```python
from build123d import *
from build123d.topology import SkipClean

# Parameters (mm, degrees)
ESQUISSE1_R        = 8
BOSS_EXTRU_1_DEPTH = 4.9
BOSS_EXTRU_2_START = 1.5
BOSS_EXTRU_2_DEPTH = 1.5
BOSS_EXTRU_3_DEPTH = 5


with BuildPart() as part:
    # Esquisse1 → Boss.-Extru.1 (new body)
    with BuildSketch(Plane.XY):
        with Locations((-10.25, -10)):
            Circle(ESQUISSE1_R)
        with BuildLine():
            Line((-5.751675839, -9.877200395), (-6.833750507, -9.782531128))
            Line((-6.833750507, -9.782531128), (-6.949445107, -9.126394451))
            Line((-6.949445107, -9.126394451), (-5.953521963, -8.661987862))
            ThreePointArc((-5.953521963, -8.661987862), (-6.006634107, -8.502052772), (-6.065697468, -8.344218516))
            Line((-6.065697468, -8.344218516), (-7.138261768, -8.631611254))
            Line((-7.138261768, -8.631611254), (-7.47139109, -8.054614344))
            Line((-7.47139109, -8.054614344), (-6.678798898, -7.262022153))
            ThreePointArc((-6.678798898, -7.262022153), (-6.782621037, -7.131675902), (-6.891198054, -7.005263035))
            Line((-6.891198054, -7.005263035), (-7.818046533, -7.654249327))
            Line((-7.818046533, -7.654249327), (-8.328430264, -7.225986526))
            Line((-8.328430264, -7.225986526), (-7.847635402, -6.194918616))
            ThreePointArc((-7.847635402, -6.194918616), (-7.988951343, -6.109285545), (-8.133315872, -6.028898352))
            Line((-8.133315872, -6.028898352), (-8.791112727, -6.968329619))
            Line((-8.791112727, -6.968329619), (-9.417191057, -6.740455742))
            Line((-9.417191057, -6.740455742), (-9.317216173, -5.597737589))
            ThreePointArc((-9.317216173, -5.597737589), (-9.478728542, -5.566588183), (-9.641271425, -5.541362369))
            Line((-9.641271425, -5.541362369), (-9.940094206, -6.656584169))
            Line((-9.940094206, -6.656584169), (-10.606352849, -6.656584169))
            Line((-10.606352849, -6.656584169), (-10.903477232, -5.547700874))
            ThreePointArc((-10.903477232, -5.547700874), (-11.065761738, -5.574558464), (-11.226956242, -5.607329229))
            Line((-11.226956242, -5.607329229), (-11.126406846, -6.756614081))
            Line((-11.126406846, -6.756614081), (-11.752485176, -6.984487958))
            Line((-11.752485176, -6.984487958), (-12.406540122, -6.050400691))
            ThreePointArc((-12.406540122, -6.050400691), (-12.550096477, -6.132241451), (-12.690551241, -6.219297732))
            Line((-12.690551241, -6.219297732), (-12.206963835, -7.256354271))
            Line((-12.206963835, -7.256354271), (-12.717347566, -7.684617071))
            Line((-12.717347566, -7.684617071), (-13.638885709, -7.039349117))
            ThreePointArc((-13.638885709, -7.039349117), (-13.74618945, -7.166864047), (-13.848697947, -7.298264801))
            Line((-13.848697947, -7.298264801), (-13.051434053, -8.095528695))
            Line((-13.051434053, -8.095528695), (-13.384563375, -8.672525605))
            Line((-13.384563375, -8.672525605), (-14.450903238, -8.3868007))
            ThreePointArc((-14.450903238, -8.3868007), (-14.508366703, -8.545244687), (-14.559856563, -8.705729393))
            Line((-14.559856563, -8.705729393), (-13.557961929, -9.172920534))
            Line((-13.557961929, -9.172920534), (-13.673656528, -9.829057211))
            Line((-13.673656528, -9.829057211), (-14.74934404, -9.923167674))
            ThreePointArc((-14.74934404, -9.923167674), (-14.749021481, -10.093838761), (-14.74222728, -10.264374865))
            Line((-14.74222728, -10.264374865), (-13.665452724, -10.358580432))
            Line((-13.665452724, -10.358580432), (-13.549758125, -11.014717109))
            Line((-13.549758125, -11.014717109), (-14.506309194, -11.460764198))
            ThreePointArc((-14.506309194, -11.460764198), (-14.447094307, -11.623083293), (-14.381691786, -11.78300953))
            Line((-14.381691786, -11.78300953), (-13.360941463, -11.509500306))
            Line((-13.360941463, -11.509500306), (-13.027812142, -12.086497216))
            Line((-13.027812142, -12.086497216), (-13.758807936, -12.817493011))
            ThreePointArc((-13.758807936, -12.817493011), (-13.646852578, -12.951506829), (-13.529782028, -13.081076086))
            Line((-13.529782028, -13.081076086), (-12.681156698, -12.486862233))
            Line((-12.681156698, -12.486862233), (-12.170772967, -12.915125033))
            Line((-12.170772967, -12.915125033), (-12.600738895, -13.837189942))
            ThreePointArc((-12.600738895, -13.837189942), (-12.448909121, -13.926168447), (-12.293716433, -14.009142444))
            Line((-12.293716433, -14.009142444), (-11.708090504, -13.172781941))
            Line((-11.708090504, -13.172781941), (-11.082012174, -13.400655818))
            Line((-11.082012174, -13.400655818), (-11.169878896, -14.404977051))
            ThreePointArc((-11.169878896, -14.404977051), (-10.996236031, -14.437694422), (-10.821442589, -14.463569577))
            Line((-10.821442589, -14.463569577), (-10.559109026, -13.48452739))
            Line((-10.559109026, -13.48452739), (-9.892850383, -13.48452739))
            Line((-9.892850383, -13.48452739), (-9.632173683, -14.457386077))
            ThreePointArc((-9.632173683, -14.457386077), (-9.45766281, -14.42969545), (-9.284373537, -14.395175256))
            Line((-9.284373537, -14.395175256), (-9.372796385, -13.384497479))
            Line((-9.372796385, -13.384497479), (-8.746718055, -13.156623602))
            Line((-8.746718055, -13.156623602), (-8.164782025, -13.987714383))
            ThreePointArc((-8.164782025, -13.987714383), (-8.010469052, -13.903139907), (-7.859580663, -13.812596936))
            Line((-7.859580663, -13.812596936), (-8.292239396, -12.884757289))
            Line((-8.292239396, -12.884757289), (-7.781855665, -12.456494489))
            Line((-7.781855665, -12.456494489), (-6.938532496, -13.046995729))
            ThreePointArc((-6.938532496, -13.046995729), (-6.822819391, -12.916236114), (-6.712266113, -12.78108593))
            Line((-6.712266113, -12.78108593), (-7.447769178, -12.045582865))
            Line((-7.447769178, -12.045582865), (-7.114639857, -11.468585954))
            Line((-7.114639857, -11.468585954), (-6.100183444, -11.740408731))
            ThreePointArc((-6.100183444, -11.740408731), (-6.036436962, -11.579837499), (-5.978900904, -11.416937723))
            Line((-5.978900904, -11.416937723), (-6.941241303, -10.968191026))
            Line((-6.941241303, -10.968191026), (-6.825546704, -10.312054348))
            Line((-6.825546704, -10.312054348), (-5.755303948, -10.21842024))
            ThreePointArc((-5.755303948, -10.21842024), (-5.750254354, -10.04784472), (-5.751675839, -9.877200395))
        make_face(mode=Mode.SUBTRACT)
    extrude(amount=-BOSS_EXTRU_1_DEPTH)

    # Esquisse2 → Boss.-Extru.2 (add)
    with SkipClean():  # the faces are left unmerged after this step: merging them gives an invalid solid
        with BuildSketch(Plane.XY.offset(BOSS_EXTRU_2_START)):
            with BuildLine():
                Line((-14.148674299, -16.985723922), (-136.398842928, 51.241076313))
                ThreePointArc((-136.398842928, 51.241076313), (-139.48589255, 62.125474534), (-128.601494329, 65.212524157))
                Line((-128.601494329, 65.212524157), (-6.351325701, -3.014276078))
                ThreePointArc((-6.351325701, -3.014276078), (-3.264276078, -13.898674299), (-14.148674299, -16.985723922))
            make_face()
        extrude(amount=-BOSS_EXTRU_2_DEPTH)
    add(part.part.scale(1), mode=Mode.REPLACE)  # the faces are merged on a copy

    # Esquisse3 → Boss.-Extru.3 (add)
    with BuildSketch(Plane(origin=(0, 0, 0), x_dir=(-1, 0, 0), z_dir=(0, 0, -1))):
        with BuildLine():
            ThreePointArc((136.398842928, 51.241076313), (139.48589255, 62.125474534), (128.601494329, 65.212524157))
            Line((128.601494329, 65.212524157), (91.708785743, 44.623010972))
            ThreePointArc((91.708785743, 44.623010972), (94.95190255, 37.271425877), (99.506134342, 30.651563128))
            Line((99.506134342, 30.651563128), (136.398842928, 51.241076313))
        make_face()
    extrude(amount=BOSS_EXTRU_3_DEPTH)


solid = part.part
```
Here's how the part is built. I have some questions about the finished solid (model axes, mm). A direction names the side the tool comes from. Give positions to 0.01 mm unless a question says otherwise; leave off trailing zeros. Loops run counter-clockwise (first coordinate to the right, second up) from the corner with the lowest first, then second, coordinate; pieces in that order, holes last. Notation, with made-up numbers: M 71,50 L 93,50 A18 ccw 93,85 Z; hole C -19,4.25 d10. An arc over 180 degrees is marked long. Put each result on its own line as item: value. Start each with the question number.
(1) For faces 4 (the cylindrical face through (-94.897, 37.37, -2.465)), 5 (the flat face through (-116, 49, -5)), which set-ups out of +Z, -Z, +X, -X, +Y, -Y let a thin tool reach every point of the face, with its end or its side?
(2) Will these pins go through, and if not, where does the flat tip stop? pin 1 Ø1.5 at (y, z) = (37.5, -3.5) entering from -X; pin 2 Ø13 at (x, y) = (-9, -14) entering from -Z; pin 3 Ø4 at (x, y) = (-45.5, -1.5) entering from -Z.
(3) I want a section at D-D on x = -77. Please give me the cut outline in (y, z).
(4) I want a section at A-A on z = -3.25. State how many separate pieces and enclosed holes the cut face has, then the cut area to 3 significant figures.
(5) If we mould it in two halves opening along Y, with no side actions, what happens to faces 1 (the flat face through (-10, -10, 0)), 2 (the cylindrical face through (-139.57, 61.97, -1.7)), 3 (the flat face through (-71, 21, 1.5))? For each: +Y half, -Y half, draft (parallel to the pull), parting line (faces both ways), or undercut.
(6) I need wall thicknesses on line 1 along Z through (x, y) = (-55.5, 12.5); line 2 along Y through (x, z) = (-102, -4); line 3 along Y through (x, z) = (-11, 0.75). Which ranges of each line are inside material? Lowest first, please. Write a range as [from, to].
(7) I want a section at B-B on y = 54. Please give me the cut outline in (x, z).
(8) I want a section at C-C on x = -107. Please give me the cut outline in (y, z), then the cut area to 3 significant figures.
Answer block:
1. face 4: -Z, +X, -Y
1. face 5: -Z, +X, -X, +Y, -Y
2. pin 1: x = -113.12
2. pin 2: z = -4.9
2. pin 3: z = 0
3. outline: M 18.09,0 L 36.41,0 L 36.41,1.5 L 18.09,1.5 Z
4. separate pieces: 2
4. enclosed holes: 1
4. area: 940 mm^2
5. face 1: undercut
5. face 2: parting line
5. face 3: draft
6. line 1: [0, 1.5]
6. line 2: [32.04, 50.37]
6. line 3: [-17.96, -0.42]
7. outline: M -139.29,-5 L -108.51,-5 L -108.51,1.5 L -139.29,1.5 Z
8. outline: M 34.83,-5 L 53.16,-5 L 53.16,1.5 L 34.83,1.5 Z
8. area: 119 mm^2
